Autodesk Inventor part; units mm, degrees
ref_plane "YZ Plane" through (0, 0, 0) normal (1, 0, 0) x (0, 1, 0)
ref_plane "XZ Plane" through (0, 0, 0) normal (0, 1, 0) x (-1, 0, 0)
ref_plane "XY Plane" through (0, 0, 0) normal (0, 0, 1) x (1, 0, 0)
sketch "Sketch1" plane through (0, 0, 0) normal (1, 0, 0) x (0, 1, 0)
  line L0 (19.05, 25.4) -> (-19.05, 25.4)
  line L1 (-19.05, 25.4) -> (-19.05, -25.4)
  line L2 (-19.05, -25.4) -> (19.05, -25.4)
  line L3 (19.05, -25.4) -> (19.05, 25.4)
  line L4 (19.05, 25.4) -> (-19.05, -25.4) construction
  line L5 (-19.05, 25.4) -> (19.05, -25.4) construction
  point P0 (0, 0)
  dimension "d0" = 38.1
  dimension "d1" = 50.8
extrude "Extrusion1" add sketch "Sketch1" along normal blind 6.35
sketch "Sketch2" plane through (6.35, 0, 0) normal (1, 0, 0) x (0, 0, -1)
  line L0 (25.4, 19.05) -> (-25.4, 19.05) construction
  line L1 (25.4, -19.05) -> (25.4, 19.05) construction
  point P0 (0, 0)
  point P1 (12.7, 12.954)
  point P2 (12.7, 0.254)
  point P3 (12.7, -9.271)
  dimension "d4" = 12.7
  dimension "d5" = 9.525
  dimension "d6" = 6.096
  dimension "d7" = 12.7
hole "Hole1" at (6.35, 12.954, -12.7) at (6.35, 0.254, -12.7) direction (-1, 0, 0) diameter 5.1054 end through all
hole "Hole2" at (6.35, -9.271, -12.7) direction (-1, 0, 0) diameter 3.9624 end through all
sketch "Sketch3" plane through (6.35, 0, 0) normal (1, 0, 0) x (0, 0, -1)
  line L0 (-25.4, 19.05) -> (-25.4, -19.05) construction
  point P0 (0, 0)
  point P1 (-12.7, 0)
  dimension "d22" = 12.7
hole "Hole3" at (6.35, 0, 12.7) direction (-1, 0, 0) diameter 4.9784 end through all
fillet "Fillet1" radius 6.604 4 edges at (3.175, 19.05, 25.4) (3.175, 19.05, -25.4) (3.175, -19.05, -25.4) (3.175, -19.05, 25.4)
properties part number "EL2-028" material "Aluminum 6061"
Geometry check sheet. Reference: the model listing, model coordinates, mm. Give positions to 0.01 mm unless a question says otherwise; leave off trailing zeros. Order: outer loops, then holes, each group sorted by start corner. A loop starts at its lowest first (then second) coordinate and runs counter-clockwise, first axis right, second up. Notation, with made-up numbers: (-29, 62) -> (4, 62) arc R12 cw to (4, 75) -> close; hole circle Ø11 at (20.25, -28.5). An arc over 180 degrees is marked (long way). Write each question's results on one line, items separated by ' | '. Start each with the question number.
(1) Scan lines: line 1 (Z direction, x = 3, y = 0); line 2 (Y direction, x = 1.75, z = -12.7); line 3 (Z direction, x = 0.5, y = -0.5). Record each from-to range of solid material in increasing order.
(2) Mould release check, pull along Z, two halves, no side actions. Record for faces 1 (the face through (3, -19.05, 0)), 2 (the face through (3.13, 1.23, -15.06)), 3 (the face through (3, 0, 25.4)): pulls with the +Z half, pulls with the -Z half, needs draft (parallel to the pull), parting line crosses it, or undercut.
(3) Sectioned sample at B-B (z = -12.7). Enter the section's corners in (x, y).
(4) Sectioned sample at A-A (z = 12.7). Enter the section's corners in (x, y).
(5) Sectioned sample at D-D (x = 4.25). Enter the section's corners in (y, z), plus the area to 3 significant figures.
(6) Sectioned sample at C-C (y = 1). Enter the section's corners in (x, z).
(7) Gauge pin test, flat end, axial feed: P1, Ø1, axis at x = 4, z = -20, coming from the -Y side. Record the tip position at first contact, or that the pin passes through.
Answer below:
1) line 1: -25.4 to -15.24, -10.16 to 10.21, 15.19 to 25.4 | line 2: -19.05 to -11.25, -7.29 to -2.3, 2.81 to 10.4, 15.51 to 19.05 | line 3: -25.4 to -15.14, -10.26 to 10.26, 15.14 to 25.4
2) face 1: needs draft | face 2: undercut | face 3: pulls with the +Z half
3) outline: (0, -19.05) -> (6.35, -19.05) -> (6.35, -11.25) -> (0, -11.25) -> close; (0, -7.29) -> (6.35, -7.29) -> (6.35, -2.3) -> (0, -2.3) -> close; (0, 2.81) -> (6.35, 2.81) -> (6.35, 10.4) -> (0, 10.4) -> close; (0, 15.51) -> (6.35, 15.51) -> (6.35, 19.05) -> (0, 19.05) -> close
4) outline: (0, -19.05) -> (6.35, -19.05) -> (6.35, -2.49) -> (0, -2.49) -> close; (0, 2.49) -> (6.35, 2.49) -> (6.35, 19.05) -> (0, 19.05) -> close
5) outline: (-19.05, -18.8) arc R6.6 ccw to (-12.45, -25.4) -> (12.45, -25.4) arc R6.6 ccw to (19.05, -18.8) -> (19.05, 18.8) arc R6.6 ccw to (12.45, 25.4) -> (-12.45, 25.4) arc R6.6 ccw to (-19.05, 18.8) -> close; hole circle Ø3.96 at (-9.27, -12.7); hole circle Ø4.98 at (0, 12.7); hole circle Ø5.11 at (0.25, -12.7); hole circle Ø5.11 at (12.95, -12.7) | area: 1,830 mm2
6) outline: (0, -25.4) -> (6.35, -25.4) -> (6.35, -15.14) -> (0, -15.14) -> close; (0, -10.26) -> (6.35, -10.26) -> (6.35, 10.42) -> (0, 10.42) -> close; (0, 14.98) -> (6.35, 14.98) -> (6.35, 25.4) -> (0, 25.4) -> close
7) P1: y = -19.01
